Study the drawing (mm; zero at the part's minimum x, y, z) and answer. A direction names the side the tool comes from. Give positions to 0.01 mm unless a question says otherwise; leave off trailing zeros. Write each loop counter-clockwise with the first axis right and the second up, starting at its lowest first coordinate (ties: lowest second). Pieces come first, ordered by that corner, then holes. Notation, with made-up numbers: (29.25, -29.5) - (35.25, -29.5) arc R32 ccw to (35.25, 6.5) - close; hole circle Ø8 at (64.25, 77.25). An arc over 180 degrees is marked (long way). Write each question's results on one line, items separated by ' | '. Start each with the question number.
Q1. For the marked faces 1 and 2, determine the directions among +Z, -Z, +X, -X, +Y, -Y from which every point of the face is accessible in a straight line to the end or side of a thin tool.
Q2. For a pull along Z with two mould halves and no side action, classify the marked faces 3, 4 and 5 as pulls with the +Z half, pulls with the -Z half, needs draft (parallel to the pull), parting line crosses it, or undercut.
Q3. Section D-D (x = 5.25) is taken. Determine the outline of the cut face in (y, z) (3 decimals).
Q4. Section C-C (z = 17) is taken. Determine the outline of the cut face in (x, y), plus the area to 3 significant figures.
Q5. Find the intervals of material crossed by probe 1 along X at (y, z) = (9.5, 11.25); probe 2 along Y at (x, z) = (3, 12.7) (3 decimals); probe 3 along Z at (x, y) = (5, 6.5), in increasing order.
Q6. Section A-A (y = 6.35) is taken. Determine the outline of the cut face in (x, z) (3 decimals), plus the area to 3 significant figures.
Q7. Section B-B (z = 12.7) is taken. Determine the outline of the cut face in (x, y) (3 decimals), plus the area to 3 significant figures.
Q8. Flat-ended cylindrical pins translate along their axes: pin 1 Ø5 at (y, z) = (6.35, 12.7) entering from -X; pin 2 Ø1.9 at (x, y) = (9, 8) entering from -Z. Find the tip coordinate at first contact, or state that the pin passes through.
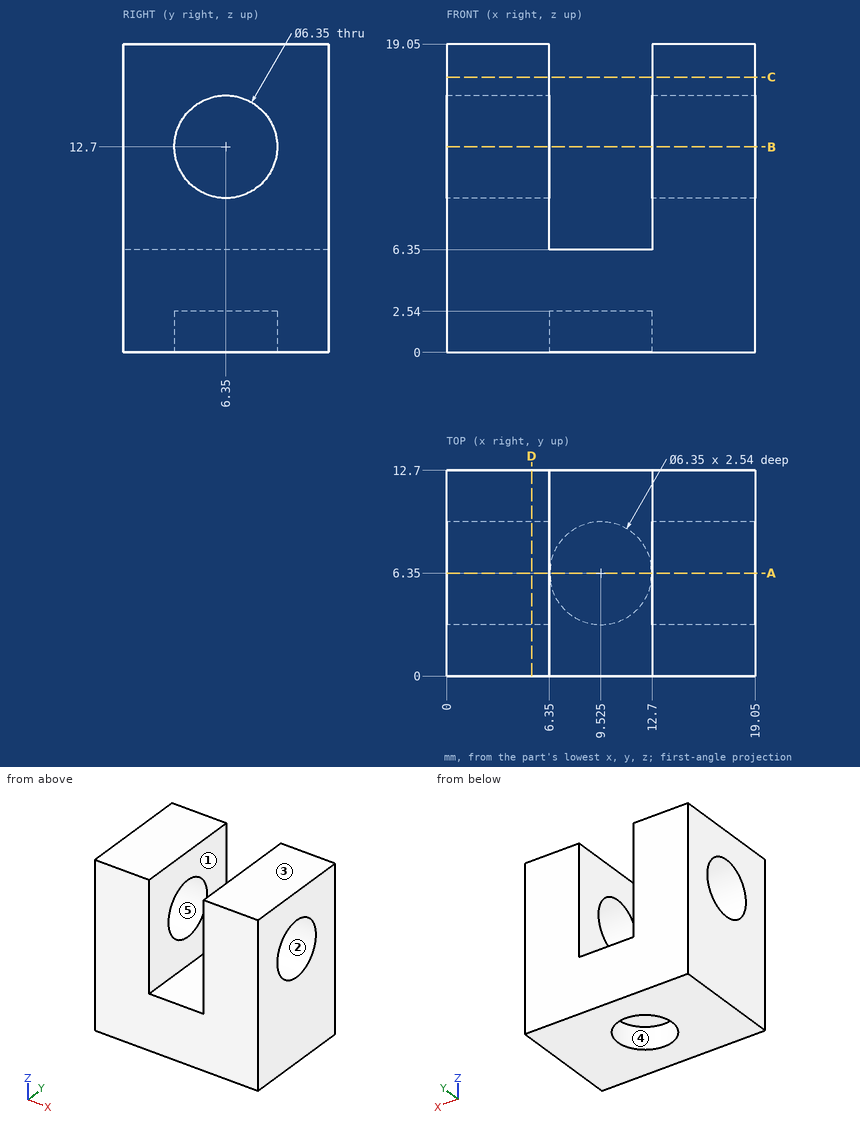
Answers below:
1) face 1: +Z, +Y, -Y | face 2: +X, -X
2) face 3: pulls with the +Z half | face 4: needs draft | face 5: undercut
3) outline: (0, 0) - (12.7, 0) - (12.7, 19.05) - (0, 19.05) - close; hole circle Ø6.35 at (6.35, 12.7)
4) outline: (0, 0) - (6.35, 0) - (6.35, 12.7) - (0, 12.7) - close; (12.7, 0) - (19.05, 0) - (19.05, 12.7) - (12.7, 12.7) - close | area: 161 mm2
5) probe 1: x = 0 to 6.35, 12.7 to 19.05 | probe 2: y = 0 to 3.175, 9.525 to 12.7 | probe 3: z = 0 to 9.53, 15.87 to 19.05
6) outline: (0, 0) - (6.35, 0) - (6.35, 2.54) - (12.7, 2.54) - (12.7, 0) - (19.05, 0) - (19.05, 9.525) - (12.7, 9.525) - (12.7, 6.35) - (6.35, 6.35) - (6.35, 9.525) - (0, 9.525) - close; (0, 15.875) - (6.35, 15.875) - (6.35, 19.05) - (0, 19.05) - close; (12.7, 15.875) - (19.05, 15.875) - (19.05, 19.05) - (12.7, 19.05) - close | area: 185 mm2
7) outline: (0, 0) - (6.35, 0) - (6.35, 3.175) - (0, 3.175) - close; (0, 9.525) - (6.35, 9.525) - (6.35, 12.7) - (0, 12.7) - close; (12.7, 0) - (19.05, 0) - (19.05, 3.175) - (12.7, 3.175) - close; (12.7, 9.525) - (19.05, 9.525) - (19.05, 12.7) - (12.7, 12.7) - close | area: 80.6 mm2
8) pin 1: passes through | pin 2: stops at z = 2.54
